```python
from build123d import *

# Parameters (mm, degrees)
SKETCH1_W           = 457.2
SKETCH1_H           = 457.2
BOSS_EXTRUDE1_DEPTH = 12.7
SKETCH2_W           = 279.4
SKETCH2_H           = 279.4
CUT_EXTRUDE1_DEPTH  = 324.538575753
SKETCH3_W           = 12.7
SKETCH3_H           = 12.7
SKETCH3_W_2         = 63.5
SKETCH3_H_2         = 63.5
SKETCH3_W_3         = 76.2
SKETCH3_H_3         = 76.2
CUT_EXTRUDE2_DEPTH  = 324.538575753


with BuildPart() as part:
    # Sketch1 → Boss-Extrude1 (new body)
    with BuildSketch(Plane(origin=(0, 0, 0), x_dir=(1, 0, 0), z_dir=(0, 1, 0))):
        Rectangle(SKETCH1_W, SKETCH1_H)
    extrude(amount=BOSS_EXTRUDE1_DEPTH)

    # Sketch2 → Cut-Extrude1 (cut, through all)
    with BuildSketch(Plane(origin=(0, 12.7, 0), x_dir=(1, 0, 0), z_dir=(0, 1, 0))):
        Rectangle(SKETCH2_W, SKETCH2_H)
    extrude(amount=-CUT_EXTRUDE1_DEPTH, mode=Mode.SUBTRACT)

    # Sketch3 → Cut-Extrude2 (cut, through all)
    with BuildSketch(Plane(origin=(0, 12.7, 0), x_dir=(1, 0, 0), z_dir=(0, 1, 0))):
        with Locations((-222.25, 222.25)):
            Rectangle(SKETCH3_W, SKETCH3_H)
        with Locations((-184.15, 222.25)):
            Rectangle(SKETCH3_W_2, SKETCH3_H)
        with Locations((-222.25, 184.15)):
            Rectangle(SKETCH3_W, SKETCH3_H_2)
        with Locations((-38.1, 222.25)):
            Rectangle(SKETCH3_W_3, SKETCH3_H)
        with Locations((114.3, 222.25)):
            Rectangle(SKETCH3_W_3, SKETCH3_H)
        with Locations((222.25, -222.25)):
            Rectangle(SKETCH3_W, SKETCH3_H)
        with Locations((184.15, -222.25)):
            Rectangle(SKETCH3_W_2, SKETCH3_H)
        with Locations((222.25, -184.15)):
            Rectangle(SKETCH3_W, SKETCH3_H_2)
        with Locations((222.25, -38.1)):
            Rectangle(SKETCH3_W, SKETCH3_H_3)
        with Locations((222.25, 114.3)):
            Rectangle(SKETCH3_W, SKETCH3_H_3)
        with Locations((38.1, -222.25)):
            Rectangle(SKETCH3_W_3, SKETCH3_H)
        with Locations((-114.3, -222.25)):
            Rectangle(SKETCH3_W_3, SKETCH3_H)
        with Locations((-222.25, 38.1)):
            Rectangle(SKETCH3_W, SKETCH3_H_3)
        with Locations((-222.25, -114.3)):
            Rectangle(SKETCH3_W, SKETCH3_H_3)
    extrude(amount=-CUT_EXTRUDE2_DEPTH, mode=Mode.SUBTRACT)


solid = part.part
```
Model file for the job. Use its own axes, mm. A direction names the side the tool comes from. Coordinates: 2 decimals unless noted, no trailing zeros. Write each loop counter-clockwise with the first axis right and the second up, starting at its lowest first coordinate (ties: lowest second). Pieces come first, ordered by that corner, then holes. Notation, with made-up numbers: (82, 78) - (98, 78) arc R21 cw to (98, 82) - close; hole circle Ø8 at (37, -10.75). An arc over 180 degrees is marked (long way). One line per question, with ' | ' between items. Start each with the question number.
Q1. 3-axis set-ups, long thin cutter, end or side, ignore diameter. For faces 4 (the face through (-222, 6, 152.4)), 5 (the face through (-76.2, 6, -222)), 6 (the face through (152.4, 6, 222)), 7 (the face through (222, 6, -152.4)), 8 (the face through (-115, 6, 215.9)): which of +Z, -Z, +X, -X, +Y, -Y reach the whole face in a straight line?
Q2. Cut at A-A, the plane z = 134.5. List the corners of the cut face in (x, y), then the cut area to 3 significant figures.
Q3. Pin check, flat tips, straight feed: pin 1 (6.5 mm diameter, centred on x = 220, y = 5.5, fed in from +Z); pin 2 (4 mm diameter, centred on y = 3.5, z = 224, fed in from +X); pin 3 (6.5 mm diameter, centred on y = 9.5, z = -54, fed in from -X). Stop position of each tip, or through.
Q4. Pull direction Z, two halves, no side cores. Call faces 1 (the face through (-222, 6, 0)), 2 (the face through (-39, 6, -215.9)), 3 (the face through (-228.6, 6, -114)): pulls with the +Z half, pulls with the -Z half, needs draft (parallel to the pull), parting line crosses it, or undercut.
Q5. Cut at C-C, the plane z = -187.5. List the corners of the cut face in (x, y).
Q6. Cut at B-B, the plane x = -108.5. List the corners of the cut face in (y, z).
Q7. Drill centre lines: line 1 (X direction, y = 8.25, z = 89); line 2 (X direction, y = 7.75, z = -125.5). Where is each one in solid material? Low to high. Write a range as [from, to].
Answer below:
1) face 4: -X, +Y, -Y | face 5: -Z, +Y, -Y | face 6: +Z, +X, +Y, -Y | face 7: +X, +Y, -Y | face 8: +Z, +Y, -Y
2) outline: (-215.9, 0) - (-139.7, 0) - (-139.7, 12.7) - (-215.9, 12.7) - close; (139.7, 0) - (228.6, 0) - (228.6, 12.7) - (139.7, 12.7) - close | area: 2,100 mm^2
3) pin 1: z = 152.4 | pin 2: x = 152.4 | pin 3: x = -215.9
4) face 1: undercut | face 2: pulls with the -Z half | face 3: needs draft
5) outline: (-215.9, 0) - (228.6, 0) - (228.6, 12.7) - (-215.9, 12.7) - close
6) outline: (0, -228.6) - (12.7, -228.6) - (12.7, -139.7) - (0, -139.7) - close; (0, 139.7) - (12.7, 139.7) - (12.7, 215.9) - (0, 215.9) - close
7) line 1: [-215.9, -139.7], [139.7, 228.6] | line 2: [-228.6, -139.7], [139.7, 215.9]
